For this review, use the dimensioned drawing (mm, ordinates from the lowest corner) and the shaded views. A direction names the side the tool comes from. Round coordinates to 2 decimals unless told otherwise and drop trailing zeros. Write each loop counter-clockwise with the first axis right and the second up, starting at its lowest first coordinate (ties: lowest second). Pieces come first, ordered by that corner, then holes. Notation, with made-up numbers: M 17.25,59.25 L 24.25,59.25 A23 ccw 24.25,78.25 Z; hole C 55,4.5 d6. An arc over 180 degrees is marked long. Answer in a Markdown table with one row per item.
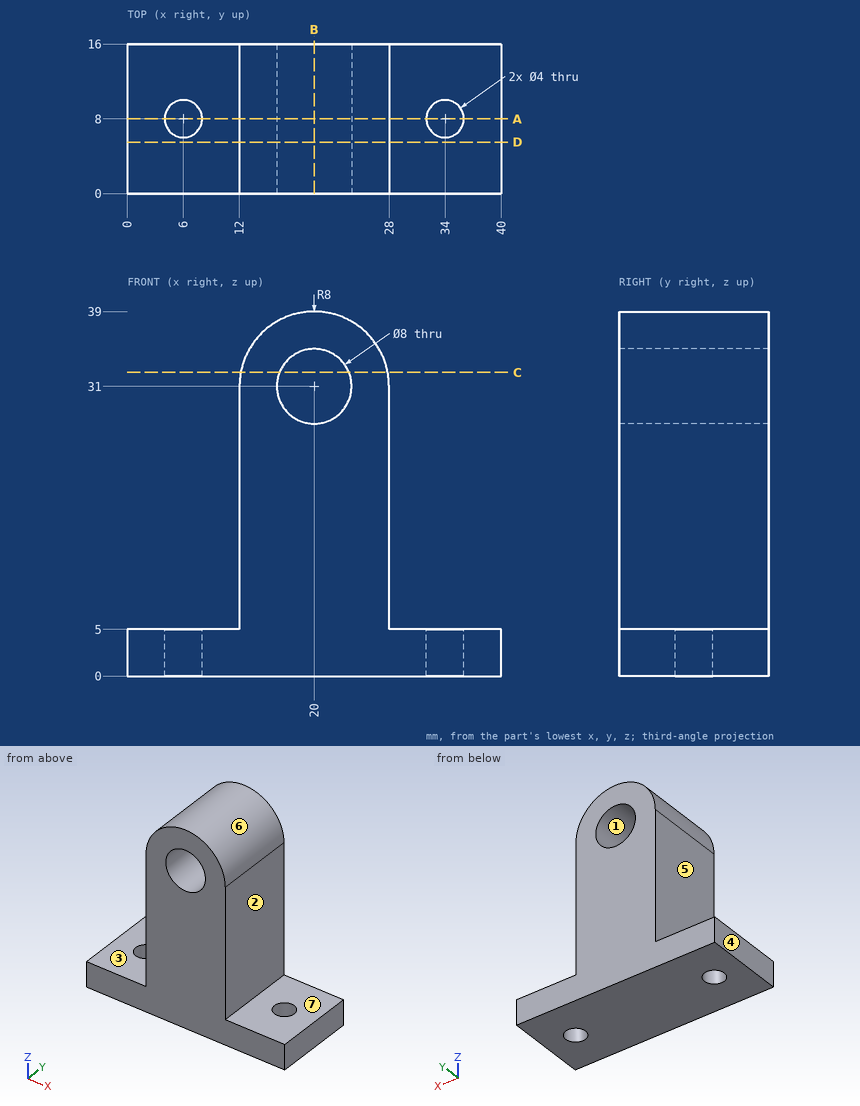
Q1. Take a section at A-A (y = 8). State the section outline as (x, z) points, then the cut area to 3 significant figures.
Found:
| item | result |
|---|---|
| outline | M 0,0 L 4,0 L 4,5 L 0,5 Z; M 8,0 L 32,0 L 32,5 L 28,5 L 28,31 A8 ccw 12,31 L 12,5 L 8,5 Z; M 36,0 L 40,0 L 40,5 L 36,5 Z; hole C 20,31 d8 |
| area | 626 mm² |
Q2. Mouldability with a two-part tool opening along X and no side actions: class the marked faces 1, 2, 3 and 4 as +X half, -X half, draft (parallel to the pull), parting line (faces both ways), or undercut.
Found:
| item | result |
|---|---|
| face 1 | undercut |
| face 2 | +X half |
| face 3 | draft |
| face 4 | -X half |
Q3. Take a section at C-C (z = 32.5). State the section outline as (x, y) points, then the cut area to 3 significant figures.
Found:
| item | result |
|---|---|
| outline | M 12.14,0 L 16.29,0 L 16.29,16 L 12.14,16 Z; M 23.71,0 L 27.86,0 L 27.86,16 L 23.71,16 Z |
| area | 133 mm² |
Q4. For probe 1 along Y at (x, z) = (34, 1.4); probe 2 along X at (y, z) = (9.5, 31); probe 3 along Z at (x, y) = (20, 4.5), list the stretches that pass through material, from the lowest coordinate up.
Found:
| item | result |
|---|---|
| probe 1 | 0 to 6, 10 to 16 |
| probe 2 | 12 to 16, 24 to 28 |
| probe 3 | 0 to 27, 35 to 39 |
Q5. Take a section at B-B (x = 20). State the section outline as (y, z) points, then the cut area to 3 significant figures.
Found:
| item | result |
|---|---|
| outline | M 0,0 L 16,0 L 16,27 L 0,27 Z; M 0,35 L 16,35 L 16,39 L 0,39 Z |
| area | 496 mm² |
Q6. Take a section at D-D (y = 5.5). State the section outline as (x, z) points, then the cut area to 3 significant figures.
Found:
| item | result |
|---|---|
| outline | M 0,0 L 40,0 L 40,5 L 28,5 L 28,31 A8 ccw 12,31 L 12,5 L 0,5 Z; hole C 20,31 d8 |
| area | 666 mm² |
Q7. Machinability: for the marked faces 5, 6 and 7, which of the approach directions +Z, -Z, +X, -X, +Y, -Y give a long, thin tool a straight path to every point of the face, cutting with its end or side? Answer none if there is none.
Found:
| item | result |
|---|---|
| face 5 | +Z, -X, +Y, -Y |
| face 6 | +Z, +Y, -Y |
| face 7 | +Z, +X, +Y, -Y |
Q8. Insertion check: P1, Ø3.5, axis at x = 32.5, y = 5.5, coming from the +Z side; P2, Ø2, axis at x = 22, y = 14, coming from the +Z side; P3, Ø8, axis at y = 4, z = 11, coming from the -X side. Each pin has a flat end and moves straight along its axis. Give the tip position at first contact, or say it passes through.
Found:
| item | result |
|---|---|
| P1 | z = 5 |
| P2 | z = 38.94 |
| P3 | x = 12 |
